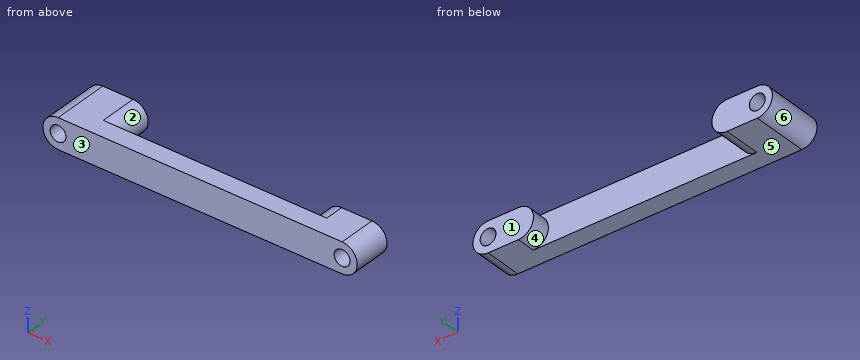
Autodesk Inventor part; units mm, degrees
ref_plane "YZ Plane" through (0, 0, 0) normal (1, 0, 0) x (0, 1, 0)
ref_plane "XZ Plane" through (0, 0, 0) normal (0, 1, 0) x (-1, 0, 0)
ref_plane "XY Plane" through (0, 0, 0) normal (0, 0, 1) x (1, 0, 0)
sketch "Sketch1" plane through (0, 0, 0) normal (0, 1, 0) x (-1, 0, 0)
  line L0 (0, 0) -> (-75.105, 0) construction
  line L1 (0, 4) -> (-75.105, 4)
  line L2 (-75.105, -4) -> (0, -4)
  arc A0 (0, -4) -> (0, 4) centre (0, 0) ccw
  arc A1 (-75.105, 4) -> (-75.105, -4) centre (-75.105, 0) ccw
  circle A2 centre (0, 0) radius 2.1
  circle A3 centre (-75.105, 0) radius 2.1
  point P0 (-37.5525, 0)
  dimension "d0" = 75.105
  dimension "d1" = 8
  dimension "d2" = 4.2
  dimension "d10" = 4.2
extrude "Extrusion1" add sketch "Sketch1" along normal blind 5
sketch "Sketch4" plane through (0, 5, 0) normal (0, 1, 0) x (1, 0, 0)
  circle A0 centre (8, 0) radius 4
  circle A1 centre (67.105, 0) radius 4
  arc A2 (75.105, -4) -> (75.105, 4) centre (75.105, 0) ccw
  line L0 (75.105, 4) -> (0, 4)
  arc A3 (0, 4) -> (0, -4) centre (0, 0) ccw
  line L1 (0, -4) -> (75.105, -4)
  circle A4 centre (75.105, 0) radius 2.1
  circle A5 centre (0, 0) radius 2.1
  point P0 (8, -4)
  point P1 (8, 4)
  point P2 (67.105, 4)
  point P3 (67.105, -4)
  dimension "d30" = 8
  dimension "d31" = 8
  dimension "d32" = 8
  dimension "d33" = 8
extrude "Extrusion7" add sketch "Sketch4" along normal blind 10 contours A0 | A0 L1 A3 L0
extrude "Extrusion8" add sketch "Sketch4" along normal blind 5 contours L0 A2 L1 A1 | A1
Could you check a few things on this model? Use its own coordinates, in mm. Face numbers are marked on the shaded views. A direction names the side the tool comes from. Coordinates: 2 decimals unless noted, no trailing zeros. Order: outer loops, then holes, each group sorted by start corner. A loop starts at its lowest first (then second) coordinate and runs counter-clockwise, first axis right, second up. Notation, with made-up numbers: M 29.25,-25 L 70.25,-25 A22 ccw 70.25,6 Z; hole C 88.5,-34.5 d10. An arc over 180 degrees is marked long. Use one line per item in the form item = value. Start each with the question number.
1. Suppose I cut it at A-A on y = 8.25. Write out the boundary of the cut face in (x, z) (3 decimals), then the cut area to 3 significant figures.
2. Suppose I cut it at C-C on z = 3. Write out the boundary of the cut face in (x, y), then the cut area to 3 significant figures.
3. On a 3-axis mill with a long thin cutter (end or side, diameter ignored), from which of +Z, -Z, +X, -X, +Y, -Y can I reach the whole of each face in a straight line? I mean the marked faces 1, 2 and 3. Say none if no direction works.
4. We'd pull the mould along X, two halves only. Please class the marked faces 4, 5 and 6: +X half, -X half, draft (parallel to the pull), parting line (faces both ways), or undercut.
5. For pin 1 (1.5 mm diameter, centred on y = 11.5, z = 1, fed in from -X); pin 2 (6 mm diameter, centred on x = 61.5, y = 10.5, fed in from -Z), each with a flat end and sliding along its axis, tell me the tip position at first contact or that it passes through.
6. Suppose I cut it at D-D on x = 13.5. Write out the boundary of the cut face in (y, z), then the cut area to 3 significant figures.
7. Please list where these lines run through material, in increasing order: line 1 (X direction, y = 2.5, z = 0) (3 decimals); line 2 (X direction, y = 5.5, z = 0) (3 decimals); line 3 (X direction, y = 4.75, z = -1).
8. Suppose I cut it at B-B on y = 3.5. Write out the boundary of the cut face in (x, z) (3 decimals).
Geometry says:
q1.outline = M 0,-4 L 8,-4 A4 ccw 8,4 L 0,4 A4 ccw Z; M 67.105,-4 L 75.105,-4 A4 ccw 75.105,4 L 67.105,4 A4 ccw Z; hole C 0,0 d4.2; hole C 75.105,0 d4.2
q1.area = 201 mm^2
q2.outline = M -2.65,0 L 77.75,0 L 77.75,10 L 64.46,10 L 64.46,5 L 10.65,5 L 10.65,15 L -2.65,15 Z
q2.area = 601 mm^2
q3.face_1 = +Z, -Z, +X, +Y
q3.face_2 = +Y
q3.face_3 = +Z, -Z, +X, -X, -Y
q4.face_4 = undercut
q4.face_5 = draft
q4.face_6 = -X half
q5.pin_1 = -3.99
q5.pin_2 = -3
q6.outline = M 0,-4 L 5,-4 L 5,4 L 0,4 Z
q6.area = 40.0 mm^2
q7.line_1 = -4 to -2.1, 2.1 to 73.005, 77.205 to 79.105
q7.line_2 = -4 to -2.1, 2.1 to 12, 63.105 to 73.005, 77.205 to 79.105
q7.line_3 = -3.87 to -1.85, 1.85 to 73.26, 76.95 to 78.98
q8.outline = M 0,-4 L 75.105,-4 A4 ccw 75.105,4 L 0,4 A4 ccw Z; hole C 0,0 d4.2; hole C 75.105,0 d4.2
